Read the model definition and answer for the solid it produces. Units are mm, in the model's axes. A direction names the side the tool comes from. Give positions to 0.01 mm unless a question says otherwise; leave off trailing zeros. Write each loop counter-clockwise with the first axis right and the second up, starting at its lowest first coordinate (ties: lowest second). Pieces come first, ordered by that corner, then holes. Notation, with made-up numbers: (32, 79) -> (45, 79) arc R26 cw to (45, 110) -> close; hole circle Ø9 at (-18.75, 13.5). An arc over 180 degrees is marked (long way). Write item = value, one per line.
from build123d import *

# Parameters (mm, degrees)
EXTRUDE1_DEPTH                                     = 60
CBORE_FOR_M3_5_PAN_HEAD_MACHINE_SCREW1_D           = 3.9
CBORE_FOR_M3_5_PAN_HEAD_MACHINE_SCREW1_CBORE_D     = 8
CBORE_FOR_M3_5_PAN_HEAD_MACHINE_SCREW1_CBORE_DEPTH = 2.6
CBORE_FOR_M4_PAN_HEAD_MACHINE_SCREW1_D             = 4.5
CBORE_FOR_M4_PAN_HEAD_MACHINE_SCREW1_CBORE_D       = 9
CBORE_FOR_M4_PAN_HEAD_MACHINE_SCREW1_CBORE_DEPTH   = 2


with BuildPart() as part:
    # Sketch1 → Extrude1 (new body)
    with BuildSketch(Plane.XY):
        with BuildLine():
            Line((-22, 0), (0, 0))
            Line((0, 0), (0, -25))
            Line((0, -25), (-2, -25))
            ThreePointArc((-2, -25), (-3.414213562, -24.414213562), (-4, -23))
            Line((-4, -23), (-4, -10.5))
            ThreePointArc((-4, -10.5), (-4.878679656, -8.378679656), (-7, -7.5))
            Line((-7, -7.5), (-22, -7.5))
            ThreePointArc((-22, -7.5), (-23.414213562, -6.914213562), (-24, -5.5))
            Line((-24, -5.5), (-24, -2))
            ThreePointArc((-24, -2), (-23.414213562, -0.585786438), (-22, 0))
        make_face()
    extrude(amount=-EXTRUDE1_DEPTH)

    # CBORE for M3.5 Pan Head Machine Screw1 (through all)
    with Locations(Plane(origin=(0, 0, 0), x_dir=(0, 0, -1), z_dir=(1, 0, 0))):
        with Locations((50, -18), (30, -18), (10, -18)):
            CounterBoreHole(CBORE_FOR_M3_5_PAN_HEAD_MACHINE_SCREW1_D / 2, CBORE_FOR_M3_5_PAN_HEAD_MACHINE_SCREW1_CBORE_D / 2, CBORE_FOR_M3_5_PAN_HEAD_MACHINE_SCREW1_CBORE_DEPTH)

    # CBORE for M4 Pan Head Machine Screw1 (through all)
    with Locations(Plane(origin=(0, 0, 0), x_dir=(-1, 0, 0), z_dir=(0, 1, 0))):
        with Locations((16, -48), (16, -12)):
            CounterBoreHole(CBORE_FOR_M4_PAN_HEAD_MACHINE_SCREW1_D / 2, CBORE_FOR_M4_PAN_HEAD_MACHINE_SCREW1_CBORE_D / 2, CBORE_FOR_M4_PAN_HEAD_MACHINE_SCREW1_CBORE_DEPTH)


solid = part.part
(1) The part is cut by section B-B on y = -18. Determine the outline of the cut face in (x, z).
Checks:
outline = (-4, -60) -> (0, -60) -> (0, -54) -> (-2.6, -54) -> (-2.6, -51.95) -> (-4, -51.95) -> close; (-4, -48.05) -> (-2.6, -48.05) -> (-2.6, -46) -> (0, -46) -> (0, -34) -> (-2.6, -34) -> (-2.6, -31.95) -> (-4, -31.95) -> close; (-4, -28.05) -> (-2.6, -28.05) -> (-2.6, -26) -> (0, -26) -> (0, -14) -> (-2.6, -14) -> (-2.6, -11.95) -> (-4, -11.95) -> close; (-4, -8.05) -> (-2.6, -8.05) -> (-2.6, -6) -> (0, -6) -> (0, 0) -> (-4, 0) -> close
(2) The part is cut by section A-A on x = -16. Determine the outline of the cut face in (y, z), plus the area to 4 significant figures.
Checks:
outline = (-7.5, -60) -> (0, -60) -> (0, -52.5) -> (-2, -52.5) -> (-2, -50.25) -> (-7.5, -50.25) -> close; (-7.5, -45.75) -> (-2, -45.75) -> (-2, -43.5) -> (0, -43.5) -> (0, -16.5) -> (-2, -16.5) -> (-2, -14.25) -> (-7.5, -14.25) -> close; (-7.5, -9.75) -> (-2, -9.75) -> (-2, -7.5) -> (0, -7.5) -> (0, 0) -> (-7.5, 0) -> close
area = 364.5 mm²
(3) For a pull along Z with two mould halves and no side action, classify faces 1 (the cylindrical face through (-14.79, -4.788, -46.103)), 2 (the flat face through (-1, -25, -30)), 3 (the flat face through (-9, -7, -60)) as released by +Z, released by -Z, zero draft, split by the parting line, or undercut.
Checks:
face_1 = undercut
face_2 = zero draft
face_3 = released by -Z
(4) The part is cut by section D-D on z = -21. Determine the outline of the cut face in (x, y), plus the area to 3 significant figures.
Checks:
outline = (-24, -5.5) arc R2 ccw to (-22, -7.5) -> (-7, -7.5) arc R3 cw to (-4, -10.5) -> (-4, -23) arc R2 ccw to (-2, -25) -> (0, -25) -> (0, 0) -> (-22, 0) arc R2 ccw to (-24, -2) -> close
area = 249 mm²
(5) Given P1, Ø6, axis at y = -15, z = -23, coming from the -X side; P2, Ø10, axis at x = -15, z = -18, coming from the -Y side; P3, Ø4, axis at y = -17.5, z = -11, coming from the +X side; P4, Ø2.5, axis at y = -18, z = -30, coming from the +X side, each flat-ended and moving along its own axis, determine where each tip first touches the part or whether it passes through.
Checks:
P1 = -4
P2 = -7.5
P3 = -2.6
P4 = through
(6) The part is cut by section C-C on z = -30. Determine the outline of the cut face in (x, y).
Checks:
outline = (-24, -5.5) arc R2 ccw to (-22, -7.5) -> (-7, -7.5) arc R3 cw to (-4, -10.5) -> (-4, -16.05) -> (-2.6, -16.05) -> (-2.6, -14) -> (0, -14) -> (0, 0) -> (-22, 0) arc R2 ccw to (-24, -2) -> close; (-4, -23) arc R2 ccw to (-2, -25) -> (0, -25) -> (0, -22) -> (-2.6, -22) -> (-2.6, -19.95) -> (-4, -19.95) -> close
(7) A tool of negligible diameter and unlimited length cuts with its end or side. For faces 4 (the flat face through (-4, -15, -30)), 5 (the flat face through (-18, -2, -14)), 6 (the flat face through (-2.6, -20, -9)), from which of +Z, -Z, +X, -X, +Y, -Y can it reach the whole face along a straight path? Write none if from no direction.
Checks:
face_4 = +Z, -Z, -X, -Y
face_5 = +Y
face_6 = +X
(8) Consider L1, parallel to Z at x = -16, y = -0.7; L2, parallel to Y at x = -1.5, z = -30; L3, parallel to Y at x = -7.75, z = -53.5. Determine where each line is inside the solid, lowest interval first.
Checks:
L1 = -60 to -52.5, -43.5 to -16.5, -7.5 to 0
L2 = -25 to -22, -14 to 0
L3 = -7.5 to 0
